from build123d import *

# Parameters (mm, degrees)
F0_W        = 80
F0_H        = 80
F1_DEPTH    = 80
F2_DEPTH    = 25
F3_R        = 15
F4_DEPTH    = 105.001
F5_T1_DEPTH = 105
F5_T3_DEPTH = 105


# Not quite as in the source:
# - a fillet or chamfer that OpenCascade refuses, or shapes differently, is made with other operations: its cross-section is extruded or revolved along the edge and cut away or added


with BuildPart() as f1:
    # F0 (on Top) → F1 (new body)
    with BuildSketch(Plane.XY):
        with Locations((-101.8917422961, 32.1563994512)):
            Rectangle(F0_W, F0_H)
    extrude(amount=F1_DEPTH)

    # F2 (add): a face of the model
    f2_faces = [f1.faces().sort_by_distance(p)[0] for p in [
        (-101.8917422961, 32.1563994512, 80),
    ]]
    extrude(f2_faces, amount=F2_DEPTH)

    # F3 (on face) → F4 (cut, through all)
    with BuildSketch(Plane.XY.offset(105)):
        with Locations((-123.7266734242, 48.2279583812)):
            Circle(F3_R)
    extrude(amount=-F4_DEPTH, mode=Mode.SUBTRACT)

    # F5: fillet of radius 5 on 5 edges, made by hand

    # F5_s2 → F5_t1 (cut)
    with BuildSketch(Plane.YZ.offset(-154.3917422961)):
        with BuildLine():
            ThreePointArc((72.1563994512, 100), (70.6919333571, 103.5355339059), (67.1563994512, 105))
            Line((67.1563994512, 105), (72.1563994512, 105))
            Line((72.1563994512, 105), (72.1563994512, 100))
        make_face()
        with BuildLine():
            ThreePointArc((-2.8436005488, 105), (-6.3791344547, 103.5355339059), (-7.8436005488, 100))
            Line((-7.8436005488, 100), (-7.8436005488, 105))
            Line((-7.8436005488, 105), (-2.8436005488, 105))
        make_face()
    extrude(amount=F5_T1_DEPTH, mode=Mode.SUBTRACT)

    # F5_s4 → F5_t3 (cut)
    with BuildSketch(Plane.XZ.offset(-84.6563994512)):
        with BuildLine():
            ThreePointArc((-61.8917422961, 100), (-63.3562083901, 103.5355339059), (-66.8917422961, 105))
            Line((-66.8917422961, 105), (-61.8917422961, 105))
            Line((-61.8917422961, 105), (-61.8917422961, 100))
        make_face()
        with BuildLine():
            ThreePointArc((-136.8917422961, 105), (-140.427276202, 103.5355339059), (-141.8917422961, 100))
            Line((-141.8917422961, 100), (-141.8917422961, 105))
            Line((-141.8917422961, 105), (-136.8917422961, 105))
        make_face()
    extrude(amount=F5_T3_DEPTH, mode=Mode.SUBTRACT)

    # F5_s5 → F5_t6 (revolve, cut)
    with BuildSketch(Plane.XZ.offset(-48.2279583812)):
        with BuildLine():
            ThreePointArc((-103.7266734242, 105), (-107.2622073302, 103.5355339059), (-108.7266734242, 100))
            Line((-108.7266734242, 100), (-108.7266734242, 105))
            Line((-108.7266734242, 105), (-103.7266734242, 105))
        make_face()
    revolve(axis=Axis((-123.7266734242, 48.2279583812, 105), (0, 0, 1)), mode=Mode.SUBTRACT)


solid = f1.part
Design review of the part built by this model. Coordinates are the model's own, in mm. Give positions to 0.01 mm unless a question says otherwise; leave off trailing zeros. Write each loop counter-clockwise with the first axis right and the second up, starting at its lowest first coordinate (ties: lowest second). Pieces come first, ordered by that corner, then holes. Notation, with made-up numbers: M -31,18 L 15,18 A26 ccw 15,48 Z; hole C 66,3 d2. An arc over 180 degrees is marked long. Answer as a JSON object with one key per item and string values. Group by question number.
1) For line 1 along X through (y, z) = (39.5, 23.5); line 2 along Y through (x, z) = (-125, 97.5); line 3 along Y through (x, z) = (-112, 90), list the stretches that pass through material, from the lowest coordinate up.
2) Mouldability with a two-part tool opening along Y and no side actions: class faces 1 (the face through (-102, -7.844, 49)), 2 (the face through (-135.63, 39.1, 50.7)), 3 (the face through (-102, 33, 0)) as released by +Y, released by -Y, zero draft, split by the parting line, or undercut.
3) We need section A-A (z = 61.5). Give the boundary of the cut face in (x, y).
Answer key:
{
 "1": {"line 1": "x = -141.89 to -135.93, -111.53 to -61.89", "line 2": "y = -7.84 to 33.28, 63.17 to 72.16", "line 3": "y = -7.84 to 38.87, 57.58 to 72.16"},
 "2": {"face 1": "released by -Y", "face 2": "undercut", "face 3": "zero draft"},
 "3": {"outline": "M -141.89,-7.84 L -61.89,-7.84 L -61.89,72.16 L -141.89,72.16 Z; hole C -123.73,48.23 d30"}
}
